Answer from the drawing. Dimensions are ordinates in mm from the lowest x, y and z of the part. A direction names the side the tool comes from. Coordinates: 2 decimals unless noted, no trailing zeros. Write each loop counter-clockwise with the first axis right and the second up, starting at its lowest first coordinate (ties: lowest second). Pieces come first, ordered by that corner, then holes. Notation, with made-up numbers: (19.5, 68.5) - (59.5, 68.5) arc R12 ccw to (59.5, 79.5) - close; hole circle Ø11 at (-8.75, 72). An arc over 180 degrees is marked (long way). Answer as a JSON object with one key per item and string values. Group by question number.
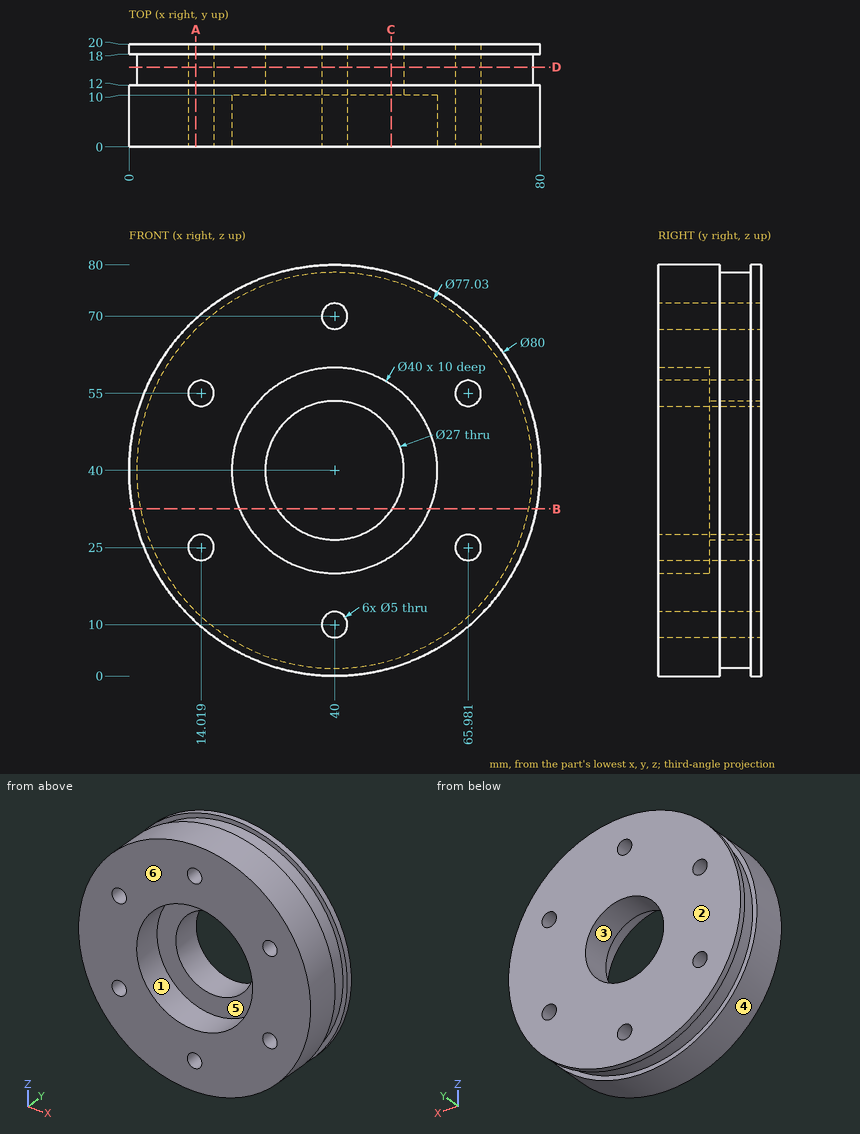
Q1. Section C-C on x = 51 is taken. Determine the outline of the cut face in (y, z).
Q2. Section B-B on z = 32.5 is taken. Determine the outline of the cut face in (x, y) (1 decimal), plus the area to 3 significant figures.
Q3. Section D-D on y = 15.5 is taken. Determine the outline of the cut face in (x, z) (1 decimal).
Q4. A tool of negligible diameter and unlimited length cuts with its end or side. For the marked faces 5 and 6, from which of +Z, -Z, +X, -X, +Y, -Y can it reach the whole face along a straight path? Write none if from no direction.
Q5. For a pull along Z with two mould halves and no side action, classify the marked faces 1, 2, 3 and 4 as +Z half, -Z half, draft (parallel to the pull), parting line (faces both ways), or undercut.
Q6. Consider L1, parallel to Z at x = 13, y = 4.5; L2, parallel to X at y = 11.25, z = 25; L3, parallel to X at y = 14, z = 40 (3 decimals). Determine where each line is inside the solid, lowest interval first. Write a range as from..to.
Q7. Section A-A on x = 13 is taken. Determine the outline of the cut face in (y, z).
Q8. Flat-ended cylindrical pins translate along their axes: pin 1 Ø1.5 at (y, z) = (6, 35) entering from -X; pin 2 Ø8 at (y, z) = (14, 44.5) entering from -X; pin 3 Ø8 at (x, z) = (40, 10) entering from -Y; pin 4 Ø6 at (x, y) = (31.5, 15.5) entering from +Z. Find the tip coordinate at first contact, or state that the pin passes through.
Numbers:
{
 "1": {"outline": "(0, 1.54) - (12, 1.54) - (12, 3.09) - (18, 3.09) - (18, 1.54) - (20, 1.54) - (20, 32.17) - (10, 32.17) - (10, 23.3) - (0, 23.3) - close; (0, 56.7) - (10, 56.7) - (10, 47.83) - (20, 47.83) - (20, 78.46) - (18, 78.46) - (18, 76.91) - (12, 76.91) - (12, 78.46) - (0, 78.46) - close"},
 "2": {"outline": "(0.7, 0) - (21.5, 0) - (21.5, 10) - (28.8, 10) - (28.8, 20) - (0.7, 20) - (0.7, 18) - (2.2, 18) - (2.2, 12) - (0.7, 12) - close; (51.2, 10) - (58.5, 10) - (58.5, 0) - (79.3, 0) - (79.3, 12) - (77.8, 12) - (77.8, 18) - (79.3, 18) - (79.3, 20) - (51.2, 20) - close", "area": "958 mm²"},
 "3": {"outline": "circle Ø77 at (40, 40); hole circle Ø5 at (14, 25); hole circle Ø5 at (14, 55); hole circle Ø27 at (40, 40); hole circle Ø5 at (40, 10); hole circle Ø5 at (40, 70); hole circle Ø5 at (66, 25); hole circle Ø5 at (66, 55)"},
 "4": {"face 5": "-Y", "face 6": "+Z, -Z, +X, -X, -Y"},
 "5": {"face 1": "undercut", "face 2": "draft", "face 3": "undercut", "face 4": "parting line"},
 "6": {"L1": "z = 10.49..22.72, 27.28..52.72, 57.28..69.51", "L2": "x = 2.92..11.52, 16.52..63.48, 68.48..77.08", "L3": "x = 1.485..26.5, 53.5..78.515"},
 "7": {"outline": "(0, 10.49) - (12, 10.49) - (12, 12.53) - (18, 12.53) - (18, 10.49) - (20, 10.49) - (20, 22.72) - (0, 22.72) - close; (0, 27.28) - (20, 27.28) - (20, 52.72) - (0, 52.72) - close; (0, 57.28) - (20, 57.28) - (20, 69.51) - (18, 69.51) - (18, 67.47) - (12, 67.47) - (12, 69.51) - (0, 69.51) - close"},
 "8": {"pin 1": "stops at x = 0.23", "pin 2": "stops at x = 0.01", "pin 3": "stops at y = 0", "pin 4": "stops at z = 79.41"}
}
